Check sheet for the modelled part. Datum: model origin and axes. Units: mm. Face numbers are marked on the shaded views. Give positions to 0.01 mm unless a question says otherwise; leave off trailing zeros. Order: outer loops, then holes, each group sorted by start corner. A loop starts at its lowest first (then second) coordinate and runs counter-clockwise, first axis right, second up.
Item 1: Material ranges on line 1 along Y through (x, z) = (17.5, 2.05); line 2 along Y through (x, z) = (5.5, 1.8); line 3 along X through (y, z) = (7.5, 2.85), recorded low to high.
Item 2: Gauge pin test, flat end, axial feed: P1, Ø2.5, axis at x = 17.5, y = 7, coming from the +Z side. Record the tip position at first contact, or that the pin passes through.
Item 3: Sectioned sample at D-D on y = 30. Record the boundary of the cut face in (x, z).
Item 4: Sectioned sample at A-A on z = 1.85. Record the boundary of the cut face in (x, y), and give its area (3 significant figures).
Item 5: Sectioned sample at C-C on x = 19. Record the boundary of the cut face in (y, z).
Item 6: Release check for a two-part mould opening along X. For the marked faces 1, 2 and 3 record: released by +X, released by -X, zero draft, split by the parting line, or undercut.
Item 7: Sectioned sample at B-B on x = 15. Record the boundary of the cut face in (y, z).
from build123d import *

# Parameters (mm, degrees)
SKETCH_1_R      = 4
SKETCH_1_R_2    = 2
EXTRUDE_1_DEPTH = 5


with BuildPart() as part:
    # 草图1 → 凸台-拉伸1 (new body)
    with BuildSketch(Plane.XY):
        with BuildLine():
            Line((2, 0), (33, 0))
            ThreePointArc((33, 0), (34.414213562, 0.585786438), (35, 2))
            Line((35, 2), (35, 21.050341825))
            Line((35, 21.050341825), (31.828098105, 38.360477291))
            ThreePointArc((31.828098105, 38.360477291), (31.141290767, 39.536384487), (29.860852284, 40))
            Line((29.860852284, 40), (5.139147716, 40))
            ThreePointArc((5.139147716, 40), (3.858709233, 39.536384487), (3.171901895, 38.360477291))
            Line((3.171901895, 38.360477291), (0, 21.050341825))
            Line((0, 21.050341825), (0, 2))
            ThreePointArc((0, 2), (0.585786438, 0.585786438), (2, 0))
        make_face()
        with Locations((17.5, 30)):
            Circle(SKETCH_1_R, mode=Mode.SUBTRACT)
        with Locations((17.5, 7)):
            Circle(SKETCH_1_R_2, mode=Mode.SUBTRACT)
        with Locations((29.5, 7)):
            Circle(SKETCH_1_R_2, mode=Mode.SUBTRACT)
        with Locations((5.5, 7)):
            Circle(SKETCH_1_R_2, mode=Mode.SUBTRACT)
    extrude(amount=EXTRUDE_1_DEPTH)


solid = part.part
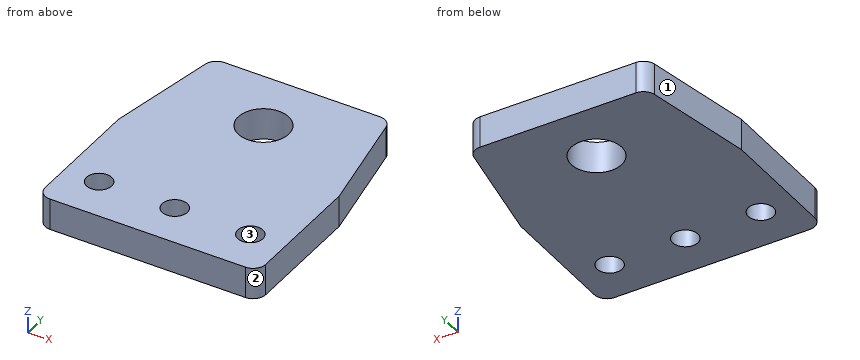
Report:
1. line 1: y = 0 to 5, 9 to 26, 34 to 40
1. line 2: y = 0 to 5, 9 to 40
1. line 3: x = 0 to 3.56, 7.44 to 15.56, 19.44 to 27.56, 31.44 to 35
2. P1: passes through
3. outline: (1.64, 0) - (13.5, 0) - (13.5, 5) - (1.64, 5) - close; (21.5, 0) - (33.36, 0) - (33.36, 5) - (21.5, 5) - close
4. outline: (0, 2) arc R2 ccw to (2, 0) - (33, 0) arc R2 ccw to (35, 2) - (35, 21.05) - (31.83, 38.36) arc R2 ccw to (29.86, 40) - (5.14, 40) arc R2 ccw to (3.17, 38.36) - (0, 21.05) - close; hole circle Ø4 at (5.5, 7); hole circle Ø8 at (17.5, 30); hole circle Ø4 at (17.5, 7); hole circle Ø4 at (29.5, 7)
4. area: 1,240 mm2
5. outline: (0, 0) - (5.68, 0) - (5.68, 5) - (0, 5) - close; (8.32, 0) - (26.29, 0) - (26.29, 5) - (8.32, 5) - close; (33.71, 0) - (40, 0) - (40, 5) - (33.71, 5) - close
6. face 1: released by -X
6. face 2: released by +X
6. face 3: undercut
7. outline: (0, 0) - (26.88, 0) - (26.88, 5) - (0, 5) - close; (33.12, 0) - (40, 0) - (40, 5) - (33.12, 5) - close
